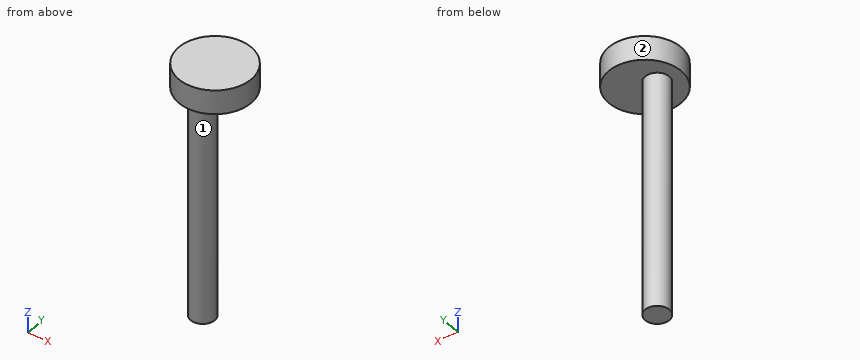
from build123d import *

# Parameters (mm, degrees)
F0_R     = 4.7625
F1_DEPTH = 80.8482
F2_R     = 14.2875
F3_DEPTH = 9.525
F4_DEPTH = 12.7


with BuildPart() as f1:
    # F0 (on Top) → F1 (new body)
    with BuildSketch(Plane.XY):
        with Locations((-7.290369, -2.118148)):
            Circle(F0_R)
    extrude(amount=F1_DEPTH)

    # F2 (on face) → F3 (join)
    with BuildSketch(Plane.XY.offset(80.8482)):
        with Locations((-2.527869, -2.118148)):
            Circle(F2_R)
    extrude(amount=F3_DEPTH)

    # F0 (on Top) → F4 (join)
    with BuildSketch(Plane.XY):
        with Locations((-7.290369, -2.118148)):
            Circle(F0_R)
    extrude(amount=-F4_DEPTH)


solid = f1.part
Build history of the part. All positions in model axes, mm. Face numbers are marked on the shaded views. A direction names the side the tool comes from. Give positions to 0.01 mm unless a question says otherwise; leave off trailing zeros. Order: outer loops, then holes, each group sorted by start corner. A loop starts at its lowest first (then second) coordinate and runs counter-clockwise, first axis right, second up. Notation, with made-up numbers: M 72,13.25 L 122,13.25 A13 cw 122,20.25 Z; hole C 2.5,49 d10. An arc over 180 degrees is marked long. Put each result on its own line as item: value.
Item 1: Slice it at D-D, the plane x = -0.5. Write the cut outline in (y, z).
From the geometry:
outline: M -16.26,80.85 L 12.02,80.85 L 12.02,90.37 L -16.26,90.37 Z
Item 2: Slice it at A-A, the plane y = -5.5. Write the cut outline in (x, z).
From the geometry:
outline: M -16.41,80.85 L -10.64,80.85 L -10.64,-12.7 L -3.94,-12.7 L -3.94,80.85 L 11.35,80.85 L 11.35,90.37 L -16.41,90.37 Z
Item 3: Probe line 1 (Z direction, x = 7, y = -3); line 2 (X direction, y = -2.25, z = 3.5); line 3 (Y direction, x = -7, z = -3). List the from-to ranges inside material, lowest first. Write a range as [from, to].
From the geometry:
line 1: z = [80.85, 90.37]
line 2: x = [-12.05, -2.53]
line 3: y = [-6.87, 2.64]
Item 4: Slice it at C-C, the plane z = 31. Write the cut outline in (x, y) (1 decimal).
From the geometry:
outline: C -7.3,-2.1 d9.5
Item 5: Flat gauge pins, fed straight in: pin 1 Ø1 at (x, y) = (-1, -5.5) entering from -Z; pin 2 Ø1 at (x, z) = (-0.5, 69) entering from +Y; pin 3 Ø12 at (y, z) = (3.5, 71) entering from -X; pin 4 Ø8 at (x, z) = (-12, 10.5) entering from +Y. Where does each tip first touch, or does it go through?
From the geometry:
pin 1: stops at z = 80.85
pin 2: passes through
pin 3: stops at x = -12.05
pin 4: stops at y = 2.59
Item 6: Slice it at B-B, the plane x = -7. Write the cut outline in (y, z).
From the geometry:
outline: M -15.69,80.85 L -6.87,80.85 L -6.87,-12.7 L 2.64,-12.7 L 2.64,80.85 L 11.45,80.85 L 11.45,90.37 L -15.69,90.37 Z
Item 7: 3-axis set-ups, long thin cutter, end or side, ignore diameter. For the marked faces 1 and 2: which of +Z, -Z, +X, -X, +Y, -Y reach the whole face in a straight line?
From the geometry:
face 1: -Z
face 2: +Z, -Z
